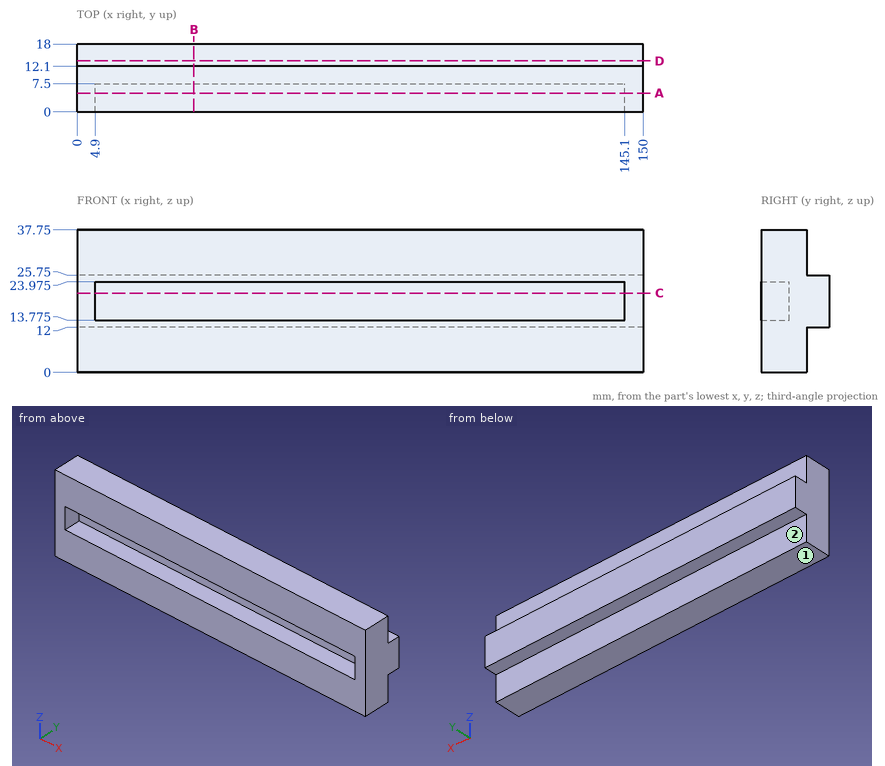
Geometry check sheet. Reference: drawing and pictorial views, mm from the part's lowest x, y, z. A direction names the side the tool comes from. Round coordinates to 2 decimals unless told otherwise and drop trailing zeros. Loops run counter-clockwise (first coordinate to the right, second up) from the corner with the lowest first, then second, coordinate; pieces in that order, holes last. Notation, with made-up numbers: (-25, 56) - (12, 56) arc R17 ccw to (12, 71) - close; hole circle Ø4 at (47.25, 48). An arc over 180 degrees is marked (long way). Use a Markdown table: item, result. Add a question column.
1. Section check C-C, the plane z = 21. Record the boundary of the cut face in (x, y).
2. Section check A-A, the plane y = 5. Record the boundary of the cut face in (x, z) (3 decimals).
3. Thickness scan on probe 1 along Z at (x, y) = (11, 6) (3 decimals); probe 2 along X at (y, z) = (1.75, 19.5); probe 3 along Z at (x, y) = (121, 13). Record the ranges inside material, lowest first. Write a range as [from, to].
4. Section check D-D, the plane y = 13.5. Record the boundary of the cut face in (x, z).
5. Section check B-B, the plane x = 31. Record the boundary of the cut face in (y, z) (3 decimals).
6. Gauge pin test, flat ends, axial feed: pin 1 (6.5 mm diameter, centred on x = 100.5, y = 16, fed in from +Z); pin 2 (8 mm diameter, centred on x = 43, z = 19.5, fed in from -Y); pin 3 (6 mm diameter, centred on x = 49, z = 7.5, fed in from +Y). Record the tip position at first contact, or that the pin passes through.
7. Access from +Z, -Z, +X, -X, +Y, -Y to the whole of each face (thin tool, end or side, straight path). Record for the marked faces 1 and 2.
Checks:
| question | item | result |
|---|---|---|
| 1 | outline | (0, 0) - (4.9, 0) - (4.9, 7.5) - (145.1, 7.5) - (145.1, 0) - (150, 0) - (150, 18) - (0, 18) - close |
| 2 | outline | (0, 0) - (150, 0) - (150, 37.75) - (0, 37.75) - close; hole (4.9, 13.775) - (145.1, 13.775) - (145.1, 23.975) - (4.9, 23.975) - close |
| 3 | probe 1 | z = [0, 13.775], [23.975, 37.75] |
| 3 | probe 2 | x = [0, 4.9], [145.1, 150] |
| 3 | probe 3 | z = [12, 25.75] |
| 4 | outline | (0, 12) - (150, 12) - (150, 25.75) - (0, 25.75) - close |
| 5 | outline | (0, 0) - (12.1, 0) - (12.1, 12) - (18, 12) - (18, 25.75) - (12.1, 25.75) - (12.1, 37.75) - (0, 37.75) - (0, 23.975) - (7.5, 23.975) - (7.5, 13.775) - (0, 13.775) - close |
| 6 | pin 1 | stops at z = 25.75 |
| 6 | pin 2 | stops at y = 7.5 |
| 6 | pin 3 | stops at y = 12.1 |
| 7 | face 1 | -Z, +X, -X, +Y, -Y |
| 7 | face 2 | -Z, +X, -X, +Y |
